For this review, take the finished solid that the model builds, in its own axes (mm). Face numbers are marked on the shaded views. A direction names the side the tool comes from. Round coordinates to 2 decimals unless told otherwise and drop trailing zeros. Order: outer loops, then holes, each group sorted by start corner. A loop starts at its lowest first (then second) coordinate and runs counter-clockwise, first axis right, second up. Notation, with made-up numbers: (47.25, 35.25) -> (66.25, 35.25) arc R7 ccw to (66.25, 42.25) -> close; hole circle Ø9 at (46.25, 70). An arc over 180 degrees is marked (long way). Use a Markdown table: item, result. Add a question column.
1) Consider section B-B (x = -10). State the section outline as (y, z) points.
2) Draft analysis for pull direction X (two halves, no side actions). For the marked faces 3, 4 and 5, state which applies: pulls with the +X half, pulls with the -X half, needs draft (parallel to the pull), parting line crosses it, or undercut.
3) Consider section A-A (y = 0). State the section outline as (x, z) points.
4) Wall thickness on line 1 along Z through (x, y) = (32.35, 0); line 2 along X through (y, z) = (-7.75, -10); line 3 along Y through (x, z) = (-6.5, 2): over which ranges is each line inside the solid? List them lowest first. Write a range as [from, to].
5) Machinability: for the marked faces 1 and 2, which of the approach directions +Z, -Z, +X, -X, +Y, -Y give a long, thin tool a straight path to every point of the face, cutting with its end or side? Answer none if there is none.
6) Clearance check with flat-ended pins moving along their axes: P1, Ø1.5, axis at x = -24, y = 8.5, coming from the +Z side; P2, Ø0.9, axis at x = -23, y = 10, coming from the -Z side; P3, Ø0.8, axis at x = 11.5, y = -12.5, coming from the +Z side. State where each tip first meets the part, or that it passes through.
7) Consider section C-C (y = -4.75). State the section outline as (x, z) points, plus the area to 3 significant figures.
8) Consider section D-D (x = 15). State the section outline as (y, z) points.
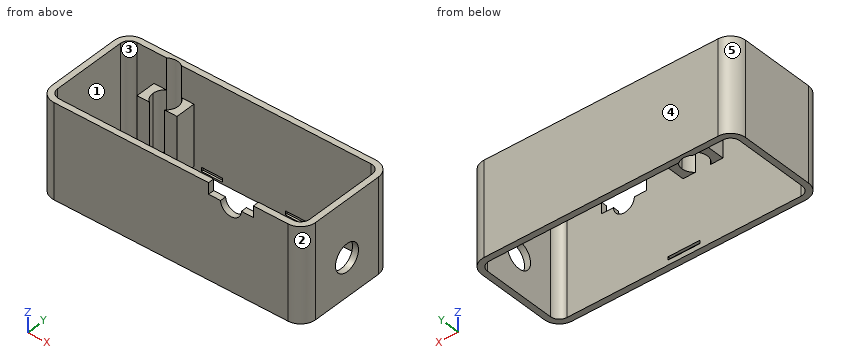
```python
from build123d import *

# Parameters (mm, degrees)
PAD_DEPTH       = 23.5
SKETCH014_W     = 8
SKETCH014_H     = 0.8
POCKET001_DEPTH = 0.7
SKETCH015_W     = 5.25
SKETCH015_H     = 1
POCKET002_DEPTH = 0.5
SKETCH020_R     = 3.4
POCKET005_DEPTH = 1.5
POCKET006_DEPTH = 1.5
SKETCH025_R     = 3.1
POCKET008_DEPTH = 23.5
PAD015_DEPTH    = 15.75
SKETCH029_W     = 10
SKETCH029_H     = 5
POCKET009_DEPTH = 0.7


with BuildPart() as part:
    # Sketch → Pad (new body)
    with BuildSketch(Plane.XY.offset(6)):
        with BuildLine():
            Line((-29.25, 13), (29.25, 13))
            ThreePointArc((33, 9.25), (31.9016504294, 11.9016504294), (29.25, 13))
            Line((33, 9.25), (33, -9.25))
            ThreePointArc((29.25, -13), (31.9016504295, -11.9016504294), (33, -9.25))
            Line((29.25, -13), (-29.25, -13))
            ThreePointArc((-33, -9.25), (-31.9016504294, -11.9016504295), (-29.25, -13))
            Line((-33, -9.25), (-33, 9.25))
            ThreePointArc((-29.25, 13), (-31.9016504294, 11.9016504294), (-33, 9.25))
        make_face()
        with BuildLine():
            Line((-29.25, 11.5), (29.25, 11.5))
            ThreePointArc((31.5, 9.25), (30.8409902577, 10.8409902577), (29.25, 11.5))
            Line((31.5, 9.25), (31.5, -9.25))
            ThreePointArc((29.25, -11.5), (30.8409902577, -10.8409902577), (31.5, -9.25))
            Line((29.25, -11.5), (-29.25, -11.5))
            ThreePointArc((-31.5, -9.25), (-30.8409902577, -10.8409902577), (-29.25, -11.5))
            Line((-31.5, -9.25), (-31.5, 9.25))
            ThreePointArc((-29.25, 11.5), (-30.8409902577, 10.8409902577), (-31.5, 9.25))
        make_face(mode=Mode.SUBTRACT)
    extrude(amount=-PAD_DEPTH)

    # Sketch014 → Pocket001 (cut)
    with BuildSketch(Plane(origin=(0, -11.5, 6), x_dir=(-1, 0, 0), z_dir=(0, 1, 0))):
        with Locations((0, -21.9)):
            Rectangle(SKETCH014_W, SKETCH014_H)
    extrude(amount=-POCKET001_DEPTH, mode=Mode.SUBTRACT)

    # Sketch015 → Pocket002 (cut)
    with BuildSketch(Plane(origin=(0, 11.5, 6), x_dir=(1, 0, 0), z_dir=(0, -1, 0))):
        with Locations((-10.475, -22.55)):
            Rectangle(SKETCH015_W, SKETCH015_H)
        with Locations((10.475, -22.55)):
            Rectangle(SKETCH015_W, SKETCH015_H)
    extrude(amount=-POCKET002_DEPTH, mode=Mode.SUBTRACT)

    # Sketch020 → Pocket005 (cut)
    with BuildSketch(Plane(origin=(33, 0, 6), x_dir=(0, 1, 0), z_dir=(1, 0, 0))):
        with Locations((0, -14)):
            Circle(SKETCH020_R)
    extrude(amount=-POCKET005_DEPTH, mode=Mode.SUBTRACT)

    # Sketch022 → Pocket006 (cut)
    with BuildSketch(Plane(origin=(0, -13, 6), x_dir=(1, 0, 0), z_dir=(0, -1, 0))):
        with BuildLine():
            ThreePointArc((12.4, -2.8), (15, -5.4), (17.6, -2.8))
            Line((17.6, -2.8), (20.6, -2.8))
            Line((20.6, -2.8), (20.6, 0.1))
            Line((9.4, 0.1), (20.6, 0.1))
            Line((9.4, -2.8), (9.4, 0.1))
            Line((12.4, -2.8), (9.4, -2.8))
        make_face()
    extrude(amount=-POCKET006_DEPTH, mode=Mode.SUBTRACT)

    # Sketch025 → Pocket008 (cut)
    with BuildSketch(Plane(origin=(0, 0, -17.5), x_dir=(1, 0, 0), z_dir=(0, 0, -1))):
        with Locations((-20, -9)):
            Circle(SKETCH025_R)
    extrude(amount=-POCKET008_DEPTH, mode=Mode.SUBTRACT)

    # Sketch026 → Pad015 (new body)
    with BuildSketch(Plane(origin=(0, 0, -17.5), x_dir=(1, 0, 0), z_dir=(0, 0, -1))):
        with BuildLine():
            Line((-15, -6.5), (-18.0836232103, -6.5))
            ThreePointArc((-16.85, -9), (-17.1751914324, -7.6061002345), (-18.0836232103, -6.5))
            ThreePointArc((-18.0836232103, -11.5), (-17.1751914324, -10.3938997655), (-16.85, -9))
            Line((-18.0836232103, -11.5), (-15, -11.5))
            Line((-15, -6.5), (-15, -11.5))
        make_face()
        with BuildLine():
            Line((-25, -11.5), (-21.9163767897, -11.5))
            ThreePointArc((-23.15, -9), (-22.8248085676, -10.3938997655), (-21.9163767897, -11.5))
            ThreePointArc((-21.9163767897, -6.5), (-22.8248085676, -7.6061002345), (-23.15, -9))
            Line((-21.9163767897, -6.5), (-25, -6.5))
            Line((-25, -6.5), (-25, -11.5))
        make_face()
    extrude(amount=-PAD015_DEPTH)

    # Sketch029 → Pocket009 (cut)
    with BuildSketch(Plane(origin=(0, 0, -17.5), x_dir=(1, 0, 0), z_dir=(0, 0, -1))):
        with Locations((-20, -9)):
            Rectangle(SKETCH029_W, SKETCH029_H)
    extrude(amount=-POCKET009_DEPTH, mode=Mode.SUBTRACT)


solid = part.part
```
Results list:
| question | item | result |
|---|---|---|
| 1 | outline | (-13, -17.5) -> (-11.5, -17.5) -> (-11.5, 6) -> (-13, 6) -> close; (11.5, -17.5) -> (13, -17.5) -> (13, 6) -> (11.5, 6) -> (11.5, -16.05) -> (12, -16.05) -> (12, -17.05) -> (11.5, -17.05) -> close |
| 2 | face 3 | undercut |
| 2 | face 4 | needs draft |
| 2 | face 5 | pulls with the -X half |
| 3 | outline | (-33, -17.5) -> (-31.5, -17.5) -> (-31.5, 6) -> (-33, 6) -> close; (31.5, -17.5) -> (33, -17.5) -> (33, -11.4) -> (31.5, -11.4) -> close; (31.5, -4.6) -> (33, -4.6) -> (33, 6) -> (31.5, 6) -> close |
| 4 | line 1 | [-17.5, -11.4], [-4.6, 6] |
| 4 | line 2 | [-33, -31.5], [31.5, 33] |
| 4 | line 3 | [-13, -11.5], [11.5, 13] |
| 5 | face 1 | +Z, -Z |
| 5 | face 2 | +Z, -Z, +X, -Y |
| 6 | P1 | z = -1.75 |
| 6 | P2 | z = -16.8 |
| 6 | P3 | z = 3.2 |
| 7 | outline | (-33, -17.5) -> (-31.5, -17.5) -> (-31.5, 6) -> (-33, 6) -> close; (31.5, -17.5) -> (33, -17.5) -> (33, 6) -> (31.5, 6) -> close |
| 7 | area | 70.5 mm2 |
| 8 | outline | (-13, -17.5) -> (-11.5, -17.5) -> (-11.5, 0.6) -> (-13, 0.6) -> close; (11.5, -17.5) -> (13, -17.5) -> (13, 6) -> (11.5, 6) -> close |
